The model under review builds one solid part; all positions refer to its coordinate system, in mm. A direction names the side the tool comes from. Coordinates: 2 decimals unless noted, no trailing zeros. Write each loop counter-clockwise with the first axis right and the second up, starting at its lowest first coordinate (ties: lowest second). Pieces come first, ordered by that corner, then holes. Notation, with made-up numbers: (-31.75, 61.25) - (20.25, 61.25) arc R8 ccw to (20.25, 68.25) - close; hole circle Ø3 at (-30.75, 44). An arc over 180 degrees is marked (long way). Answer as CSV lines item,"result". Start each with the question number.
```python
from build123d import *

# Parameters (mm, degrees)
F0_W      = 76.2
F0_H      = 58.7432836175
F0_W_2    = 12.7
F1_DEPTH  = 50.8
F3_DEPTH  = 15.24
F5_DEPTH  = 80.01
F7_DEPTH  = 25.4
F8_R      = 2.54
F10_DEPTH = 25.4
F11_W     = 43.6744932085
F11_H     = 27.1944999695
F12_DEPTH = 25.4
F14_DEPTH = 25.4


with BuildPart() as f1:
    # F0 (on Top) → F1 (new body)
    with BuildSketch(Plane.XY):
        Rectangle(F0_W, F0_H)
        with Locations((44.45, 0)):
            Rectangle(F0_W_2, F0_H)
        with Locations((-44.45, 0)):
            Rectangle(F0_W_2, F0_H)
    extrude(amount=F1_DEPTH)

    # F2 (on face) → F3 (cut)
    with BuildSketch(Plane(origin=(-50.8, 0, 0), x_dir=(0, -1, 0), z_dir=(-1, 0, 0))):
        with BuildLine():
            Line((-22.7101761848, 17.5973810256), (-22.7101761848, 0))
            Line((-22.7101761848, 0), (19.4533672184, 0))
            Line((19.4533672184, 0), (19.4533672184, 17.5973810256))
            ThreePointArc((19.4533672184, 17.5973810256), (-1.6284044832, 38.6791527271), (-22.7101761848, 17.5973810256))
        make_face()
    extrude(amount=-F3_DEPTH, mode=Mode.SUBTRACT)

    # F4 (on face) → F5 (cut)
    with BuildSketch(Plane.YZ.offset(50.8)):
        Polygon((-29.3716418087, 50.8), (-29.3716418087, 11.9435014203), (20.7798294723, 38.9182642102), (20.7798294723, 50.8), align=None)
    extrude(amount=-F5_DEPTH, mode=Mode.SUBTRACT)

    # F6 (on face) → F7 (cut)
    with BuildSketch(Plane.YZ.offset(50.8)):
        Polygon((-17.4182243645, 11.9435014203), (-17.4182243645, 0), (20.7798294723, 0), (29.3716418087, 0), (29.3716418087, 32.4889294001), (20.7798294723, 32.4889294001), align=None)
    extrude(amount=-F7_DEPTH, mode=Mode.SUBTRACT)

    # F8
    f8_edges = [f1.edges().sort_by_distance(p)[0] for p in [
        (10.795, 20.779829, 50.8),
        (-29.21, -4.295906, 50.8),
        (-40.005, -29.371642, 50.8),
        (-50.8, 0, 50.8),
        (0, 29.371642, 50.8),
        (50.8, 25.075736, 50.8),
        (-50.8, 1.628404, 38.679153),
    ]]
    fillet(f8_edges, radius=F8_R)

    # F9 (on face) → F10 (cut)
    with BuildSketch(Plane.YZ.offset(25.4)):
        Polygon((-9.3324668705, 11.9435014203), (-9.3324668705, 0), (29.3716418087, 0), (29.3716418087, 28.1398767242), (20.7798294723, 28.1398767242), align=None)
    extrude(amount=-F10_DEPTH, mode=Mode.SUBTRACT)

    # F11 (on Top) → F12 (cut)
    with BuildSketch(Plane.XY):
        with Locations((45.2370969579, 16.5996663272)):
            Rectangle(F11_W, F11_H)
    extrude(amount=-F12_DEPTH, mode=Mode.SUBTRACT)

    # F13 (on face) → F14 (cut)
    with BuildSketch(Plane.YZ):
        Polygon((-2.0139215048, 11.9435014203), (-2.0139215048, 0), (29.3716418087, 0), (29.3716418087, 24.2034812374), (20.7798294723, 24.2034812374), align=None)
    extrude(amount=-F14_DEPTH, mode=Mode.SUBTRACT)


solid = f1.part
```
(1) Add section C-C on y = -24.5. Give the boundary of the cut face in (x, z).
(2) Add section D-D on x = -4. Give the boundary of the cut face in (y, z), then the cut area to 3 significant figures.
(3) Add section B-B on z = 6.5. Give the boundary of the cut face in (x, y), then the cut area to 3 significant figures.
(4) Wall thickness on line 1 (Y direction, x = -40.5, z = 16.5); line 2 (X direction, y = -1, z = 24); line 3 (X direction, y = -11, z = 12.5): over which ranges is each line inside the solid? List them lowest first.
(5) The part is to be moulded in two halves that separate along Y. For faces 1 (the flat face through (25.4, -1, 18)), 2 (the flat face through (38.28, 1.95, 22.36)), 3 (the flat face through (-35.56, 2, 20)), say which applies: released by +Y, released by -Y, zero draft, split by the parting line, or undercut.
(6) For pin 1 (7 mm diameter, centred on x = -11.5, y = 26, fed in from -Z); pin 2 (12 mm diameter, centred on x = -7, z = 7, fed in from +Y); pin 3 (6 mm diameter, centred on x = 32.5, z = 4.5, fed in from +Y), all flat-tipped, find the tip position at first contact; note any pin that passes through.
(7) Add section A-A on x = 41. Give the boundary of the cut face in (y, z).
(8) For faces 4 (the cylindrical face through (8.947, 21.544, 50.076)), 5 (the cylindrical face through (-0.711, 28.647, 50.036)), 6 (the cylindrical face through (-50.1, 23.5, 8.7)), 7 (the flat face through (-23, -29.372, 8)), 8 (the flat face through (38, 25, 32.489)), list the 3-axis set-ups (+Z, -Z, +X, -X, +Y, -Y) from which the entire face can be reached by the end or side of a thin tool; tool diameter is ignored.
Reported:
1,outline,"(-50.8, 0) - (50.8, 0) - (50.8, 14.56) - (-29.21, 14.56) - (-29.21, 48.26) arc R2.54 ccw to (-31.75, 50.8) - (-48.26, 50.8) arc R2.54 ccw to (-50.8, 48.26) - close"
2,outline,"(-29.37, 0) - (-2.01, 0) - (-2.01, 11.94) - (20.78, 24.2) - (29.37, 24.2) - (29.37, 48.26) arc R2.54 ccw to (26.83, 50.8) - (23.32, 50.8) arc R2.54 ccw to (20.78, 48.26) - (20.78, 38.92) - (-29.37, 11.94) - close"
2,area,"1,090 mm²"
3,outline,"(-50.8, -29.37) - (50.8, -29.37) - (50.8, -17.42) - (25.4, -17.42) - (25.4, -9.33) - (0, -9.33) - (0, -2.01) - (-25.4, -2.01) - (-25.4, 29.37) - (-50.8, 29.37) - (-50.8, 25.25) arc R2.54 ccw to (-48.26, 22.71) - (-35.56, 22.71) - (-35.56, -19.45) - (-48.26, -19.45) arc R2.54 ccw to (-50.8, -21.99) - close"
3,area,"2,350 mm²"
4,line 1,"-29.37 to -19.45, 22.71 to 29.37"
4,line 2,"-35.56 to 50.8"
4,line 3,"-35.56 to 25.4"
5,face 1,"zero draft"
5,face 2,"released by +Y"
5,face 3,"undercut"
6,pin 1,"z = 24.2"
6,pin 2,"y = -0.05"
6,pin 3,"y = -17.42"
7,outline,"(-29.37, 0) - (-17.42, 0) - (-17.42, 11.94) - (20.78, 32.49) - (29.37, 32.49) - (29.37, 48.26) arc R2.54 ccw to (26.83, 50.8) - (23.32, 50.8) arc R2.54 ccw to (20.78, 48.26) - (20.78, 38.92) - (-29.37, 11.94) - close"
8,face 4,"+Z, +X, -Y"
8,face 5,"+Z, +X, -X, +Y"
8,face 6,"-Z, -X"
8,face 7,"+Z, -Z, +X, -X, -Y"
8,face 8,"-Z, +X, +Y"
